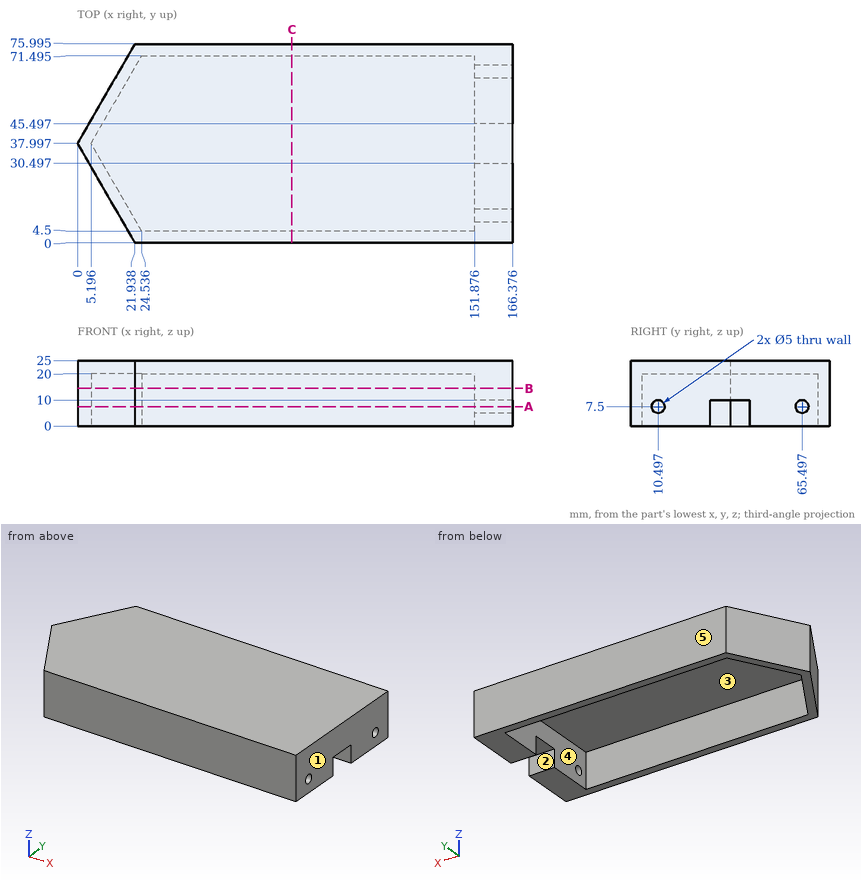
Drawing for the job (mm, zero at the part's lowest x, y, z). A direction names the side the tool comes from. Give positions to 0.01 mm unless a question says otherwise; leave off trailing zeros. Order: outer loops, then holes, each group sorted by start corner. A loop starts at its lowest first (then second) coordinate and runs counter-clockwise, first axis right, second up. Notation, with made-up numbers: M -11,-29 L 37,-29 A33 ccw 37,4 Z; hole C 23,58.25 d1. An arc over 180 degrees is marked long. Use a Markdown table: item, result. Add a question column.
(1) Drop flat-ended pins along their axis: P1, Ø5, axis at y = 62, z = 10, coming from the -X side (1 decimal); P2, Ø3, axis at y = 10.5, z = 7.5, coming from the +X side; P3, Ø11.5, axis at x = 161, y = 37.5, coming from the -Z side. Give the stop position or say it passes through.
(2) Saw through at A-A, the plane z = 7.5. Give the cut face in (x, y) (1 decimal), and give its area (3 significant figures).
(3) 3-axis set-ups, long thin cutter, end or side, ignore diameter. For the marked faces 4 and 5: which of +Z, -Z, +X, -X, +Y, -Y reach the whole face in a straight line?
(4) Mould opens along X. For the marked faces 1, 2 and 3 say: +X half, -X half, draft (parallel to the pull), parting line (faces both ways), or undercut.
(5) Probe line 1 along Y through (x, z) = (155.75, 7.5) (1 decimal); line 2 along Y through (x, z) = (60, 19.25) (1 decimal); line 3 along Z through (x, y) = (121, 21). List the from-to ranges inside material, lowest first. Write a range as [from, to].
(6) Saw through at C-C, the plane x = 82. Give the cut face in (y, z) (1 decimal), and give its area (3 significant figures).
(7) Saw through at B-B, the plane z = 14.5. Give the cut face in (x, y) (1 decimal), and give its area (3 significant figures).
Answer key:
| question | item | result |
|---|---|---|
| 1 | P1 | x = 12.4 |
| 1 | P2 | x = 21.94 |
| 1 | P3 | z = 10 |
| 2 | outline | M 0,38 L 21.9,0 L 166.4,0 L 166.4,8 L 151.9,8 L 151.9,4.5 L 24.5,4.5 L 5.2,38 L 24.5,71.5 L 151.9,71.5 L 151.9,68 L 166.4,68 L 166.4,76 L 21.9,76 Z; M 151.9,13 L 166.4,13 L 166.4,30.5 L 151.9,30.5 Z; M 151.9,45.5 L 166.4,45.5 L 166.4,63 L 151.9,63 Z |
| 2 | area | 2,270 mm^2 |
| 3 | face 4 | -Z |
| 3 | face 5 | +Z, -Z, +X, -X, +Y |
| 4 | face 1 | +X half |
| 4 | face 2 | draft |
| 4 | face 3 | undercut |
| 5 | line 1 | [0, 8], [13, 30.5], [45.5, 63], [68, 76] |
| 5 | line 2 | [0, 4.5], [71.5, 76] |
| 5 | line 3 | [20, 25] |
| 6 | outline | M 0,0 L 4.5,0 L 4.5,20 L 71.5,20 L 71.5,0 L 76,0 L 76,25 L 0,25 Z |
| 6 | area | 560 mm^2 |
| 7 | outline | M 0,38 L 21.9,0 L 166.4,0 L 166.4,76 L 21.9,76 Z; hole M 5.2,38 L 24.5,4.5 L 151.9,4.5 L 151.9,71.5 L 24.5,71.5 Z |
| 7 | area | 2,630 mm^2 |
